The listing builds one solid part. Answer for the finished solid, in the listing's coordinates (mm). Give positions to 0.01 mm unless a question says otherwise; leave off trailing zeros. Loops run counter-clockwise (first coordinate to the right, second up) from the corner with the lowest first, then second, coordinate; pieces in that order, holes last. Notation, with made-up numbers: M -10.5,36 L 6.5,36 A16 cw 6.5,50 Z; hole C 68,46 d3. An arc over 180 degrees is marked long. Use one line per item in the form item = value. Start each with the question number.
1. The part is cut by section A-A (x = 17). Write down the section's boundary in (y, z).
2. The part is cut by section D-D (z = -1.6). Give the number of separate pieces and of enclosed holes in the cut face, and give its area (3 significant figures).
3. The part is cut by section C-C (x = -16.3). Write down the section's boundary in (y, z), and give its area (3 significant figures).
4. Straight lines are drawn through the part: line 1 (Y direction, x = -16.3, z = -0.2); line 2 (Y direction, x = 8, z = -1.45); line 3 (X direction, y = 33.5, z = -1.3). For each, find the intervals that lie inside material, in ascending order. Write a range as from..to.
5. Each of these flat-tipped pins is pushed along its axis until it touches: pin 1 Ø1 at (y, z) = (19.5, 1.5) entering from +X; pin 2 Ø3 at (x, y) = (-46.63, 37.65) entering from -Z; pin 3 Ø2.5 at (y, z) = (-34, 0) entering from -X; pin 4 Ø5.5 at (x, y) = (-16.3, 24.5) entering from -Z. Where does it stop, or does it pass through?
6. The part is cut by section B-B (y = 24.5). Write down the section's boundary in (x, z), and give its area (3 significant figures).
from build123d import *

# Parameters (mm, degrees)
SKETCH1_R           = 1.800000083
SKETCH1_R_2         = 1.650000002
SKETCH1_W           = 8.89
SKETCH1_H           = 38.1
BOSS_EXTRUDE1_DEPTH = 2.54


with BuildPart() as part:
    # Sketch1 → Boss-Extrude1 (new body, symmetric)
    with BuildSketch(Plane(origin=(0, 0, 0), x_dir=(0, 1, 0), z_dir=(0, 0, 1))):
        Polygon((-41.181536726, 53.881536726), (-19.05, 53.881536726), (-12.7, 60.231536726), (12.7, 60.231536726), (19.05, 53.881536726), (41.181536726, 53.881536726), (53.881536726, 41.181536726), (53.881536726, -41.181536726), (41.181536726, -53.881536726), (19.05, -53.881536726), (12.7, -60.231536726), (-12.7, -60.231536726), (-19.05, -53.881536726), (-41.181536726, -53.881536726), (-53.881536726, -41.181536726), (-53.881536726, 41.181536726), align=None)
        with Locations((-46.633511114, -37.653254993)):
            Circle(SKETCH1_R, mode=Mode.SUBTRACT)
        with Locations((-37.653254993, -46.633511114)):
            Circle(SKETCH1_R, mode=Mode.SUBTRACT)
        with Locations((46.633511114, -37.653254993)):
            Circle(SKETCH1_R, mode=Mode.SUBTRACT)
        with Locations((37.653254993, -46.633511114)):
            Circle(SKETCH1_R, mode=Mode.SUBTRACT)
        with Locations((-46.633511114, 37.653254993)):
            Circle(SKETCH1_R, mode=Mode.SUBTRACT)
        with Locations((-37.653254993, 46.633511114)):
            Circle(SKETCH1_R, mode=Mode.SUBTRACT)
        with Locations((37.653254993, 46.633511114)):
            Circle(SKETCH1_R, mode=Mode.SUBTRACT)
        with Locations((46.633511114, 37.653254993)):
            Circle(SKETCH1_R, mode=Mode.SUBTRACT)
        with Locations((-24.5, -41.7)):
            Circle(SKETCH1_R_2, mode=Mode.SUBTRACT)
        with Locations((24.5, -41.7)):
            Circle(SKETCH1_R_2, mode=Mode.SUBTRACT)
        with Locations((24.5, 16.3)):
            Circle(SKETCH1_R_2, mode=Mode.SUBTRACT)
        with Locations((-24.5, 16.3)):
            Circle(SKETCH1_R_2, mode=Mode.SUBTRACT)
        with Locations((-9.525, -56.421536726)):
            Circle(SKETCH1_R, mode=Mode.SUBTRACT)
        with Locations((9.525, -56.421536726)):
            Circle(SKETCH1_R, mode=Mode.SUBTRACT)
        with Locations((9.525, 56.421536726)):
            Circle(SKETCH1_R, mode=Mode.SUBTRACT)
        with Locations((-9.525, 56.421536726)):
            Circle(SKETCH1_R, mode=Mode.SUBTRACT)
        with Locations((36.195, 0)):
            Rectangle(SKETCH1_W, SKETCH1_H, mode=Mode.SUBTRACT)
        with Locations((-36.195, 0)):
            Rectangle(SKETCH1_W, SKETCH1_H, mode=Mode.SUBTRACT)
    extrude(amount=BOSS_EXTRUDE1_DEPTH, both=True)


solid = part.part
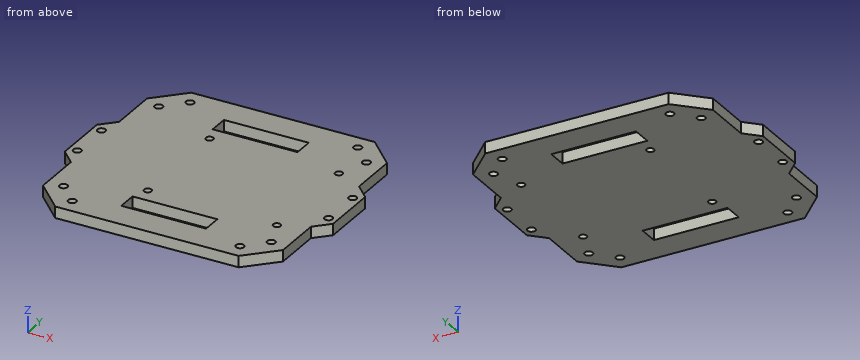
Derived:
q1.outline = M -53.88,-2.54 L -40.64,-2.54 L -40.64,2.54 L -53.88,2.54 Z; M -31.75,-2.54 L 31.75,-2.54 L 31.75,2.54 L -31.75,2.54 Z; M 40.64,-2.54 L 53.88,-2.54 L 53.88,2.54 L 40.64,2.54 Z
q2.separate_pieces = 1
q2.enclosed_holes = 18
q2.area = 10,900 mm2
q3.outline = M -53.88,-2.54 L -40.64,-2.54 L -40.64,2.54 L -53.88,2.54 Z; M -31.75,-2.54 L -26.15,-2.54 L -26.15,2.54 L -31.75,2.54 Z; M -22.85,-2.54 L 22.85,-2.54 L 22.85,2.54 L -22.85,2.54 Z; M 26.15,-2.54 L 31.75,-2.54 L 31.75,2.54 L 26.15,2.54 Z; M 40.64,-2.54 L 53.88,-2.54 L 53.88,2.54 L 40.64,2.54 Z
q3.area = 424 mm2
q4.line_1 = -53.88..-40.64, -31.75..-26.15, -22.85..22.85, 26.15..31.75, 40.64..53.88
q4.line_2 = -53.88..-40.64, -31.75..31.75, 40.64..53.88
q4.line_3 = -53.88..-19.05, 19.05..53.88
q5.pin_1 = 53.93
q5.pin_2 = through
q5.pin_3 = -53.88
q5.pin_4 = -2.54
q6.outline = M -53.88,-2.54 L -17.95,-2.54 L -17.95,2.54 L -53.88,2.54 Z; M -14.65,-2.54 L 40.05,-2.54 L 40.05,2.54 L -14.65,2.54 Z; M 43.35,-2.54 L 53.88,-2.54 L 53.88,2.54 L 43.35,2.54 Z
q6.area = 514 mm2
